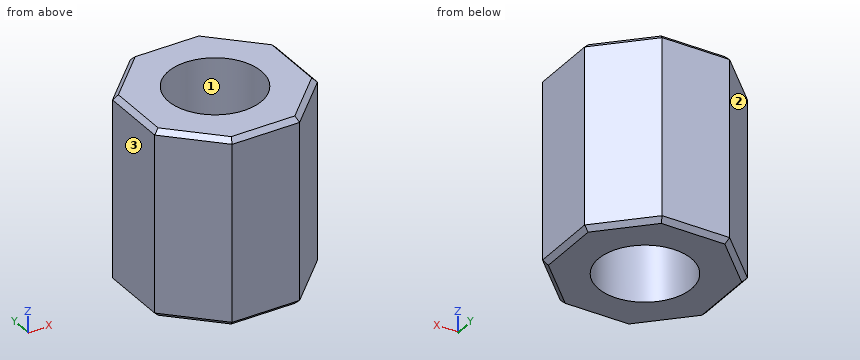
Autodesk Inventor part; units mm, degrees
ref_plane "YZ Plane" through (0, 0, 0) normal (1, 0, 0) x (0, 1, 0)
ref_plane "XZ Plane" through (0, 0, 0) normal (0, 1, 0) x (-1, 0, 0)
ref_plane "XY Plane" through (0, 0, 0) normal (0, 0, 1) x (1, 0, 0)
sketch "スケッチ1" plane through (0, 0, 0) normal (0, 0, 1) x (1, 0, 0)
  circle A0 centre (0, 0) radius 2
  arc A1 (-3.5, 0) -> (-2.4749, -2.4749) centre (0, 0) ccw
  line L0 (-3.5, 3.5) -> (3.5, 3.5)
  line L1 (3.5, 3.5) -> (3.5, -3.5)
  line L2 (3.5, -3.5) -> (-3.5, -3.5)
  line L3 (-3.5, -3.5) -> (-3.5, 3.5)
  line L4 (-4.9497, 0) -> (0, 4.9497)
  line L5 (0, -4.9497) -> (-4.9497, 0)
  line L6 (4.9497, 0) -> (0, -4.9497)
  line L7 (0, 4.9497) -> (4.9497, 0)
  line L8 (-3.5, 1.4497) -> (-1.4497, 3.5)
  line L9 (1.4497, 3.5) -> (3.5, 1.4497)
  line L10 (3.5, -1.4497) -> (1.4497, -3.5)
  line L11 (-1.4497, -3.5) -> (-3.5, -1.4497)
  point P0 (-3.5, -1.4497)
  dimension "d0" = 4
  dimension "d1" = 7
  dimension "d2" = 7
  dimension "d3" = 7
  dimension "d6" = 45
extrude "押し出し1" add sketch "スケッチ1" along normal blind 8 contours L3 L4 L0 L7 L1 L6 L2 L5 A1 | A1 L5 L3
chamfer "面取り1" distance 0.2 angle 45 8 edges at (-2.4749, 2.4749, 8) (0, 3.5, 8) (3.5, 0, 8) (0, -3.5, 8) (-2.4749, -2.4749, 8) (-3.5, 0, 8) (2.4749, 2.4749, 8) (2.4749, -2.4749, 8)
chamfer "面取り2" distance 0.2 angle 45 8 edges at (2.4749, 2.4749, 0) (3.5, 0, 0) (2.4749, -2.4749, 0) (0, 3.5, 0) (-2.4749, 2.4749, 0) (-3.5, 0, 0) (-2.4749, -2.4749, 0) (0, -3.5, 0)
properties part number "GearHub6kakku" material "アルミニウム 6061"
Input: part model. Units: mm. Frame: model coordinates. Face numbers are marked on the shaded views. Round coordinates to 2 decimals unless told otherwise and drop trailing zeros. Loops run counter-clockwise (first coordinate to the right, second up) from the corner with the lowest first, then second, coordinate; pieces in that order, holes last. Notation, with made-up numbers: (37.5, 66.5) -> (62.5, 66.5) arc R33 cw to (62.5, 104.5) -> close; hole circle Ø8 at (83, 25.5). An arc over 180 degrees is marked (long way). Answer as a JSON object with one key per item and string values. Group by question number.
1) Ray query, L1, parallel to Y at x = 0, z = 4.5; L2, parallel to X at y = 1, z = 0.75; L3, parallel to Y at x = -1.5, z = 7. Return the intervals inside material, ascending.
2) Section query A-A on y = 0. Output: boundary loops of the cut face in (x, z), plus the area to 3 significant figures.
3) Section query C-C on z = 6.75. Output: boundary loops of the cut face in (x, y), plus the area to 3 significant figures.
4) Section query D-D on y = 3. Output: boundary loops of the cut face in (x, z).
5) Pin query (flat end, axial travel): pin 1 (3.5 mm diameter, centred on x = 0, y = 0, fed in from +Z); pin 2 (1 mm diameter, centred on y = -2.5, z = 4, fed in from -X). Return the tip coordinate at first contact, or that it passes through.
6) Draft query along Y for the marked faces 1, 2 and 3. Return one class per face: +Y half, -Y half, draft (parallel to the pull), parting line (faces both ways), or undercut.
Reply:
{
 "1": {"L1": "y = -3.5 to -2, 2 to 3.5", "L2": "x = -3.5 to -1.73, 1.73 to 3.5", "L3": "y = -3.45 to -1.32, 1.32 to 3.45"},
 "2": {"outline": "(-3.5, 0.2) -> (-3.3, 0) -> (-2, 0) -> (-2, 8) -> (-3.3, 8) -> (-3.5, 7.8) -> close; (2, 0) -> (3.3, 0) -> (3.5, 0.2) -> (3.5, 7.8) -> (3.3, 8) -> (2, 8) -> close", "area": "23.9 mm2"},
 "3": {"outline": "(-3.5, -1.45) -> (-1.45, -3.5) -> (1.45, -3.5) -> (3.5, -1.45) -> (3.5, 1.45) -> (1.45, 3.5) -> (-1.45, 3.5) -> (-3.5, 1.45) -> close; hole circle Ø4 at (0, 0)", "area": "28.0 mm2"},
 "4": {"outline": "(-1.95, 0.2) -> (-1.67, 0) -> (1.67, 0) -> (1.95, 0.2) -> (1.95, 7.8) -> (1.67, 8) -> (-1.67, 8) -> (-1.95, 7.8) -> close"},
 "5": {"pin 1": "passes through", "pin 2": "stops at x = -2.95"},
 "6": {"face 1": "undercut", "face 2": "+Y half", "face 3": "draft"}
}
